Verification items for this drawing (mm, ordinates from the low corner). A direction names the side the tool comes from. Coordinates: 2 decimals unless noted, no trailing zeros. Write each loop counter-clockwise with the first axis right and the second up, starting at its lowest first coordinate (ties: lowest second). Pieces come first, ordered by that corner, then holes. Notation, with made-up numbers: (87, 87.25) -> (129, 87.25) arc R8 cw to (129, 96.25) -> close; hole circle Ø8 at (78.25, 31.25). An arc over 180 degrees is marked (long way). One line per question, with ' | ' between items.
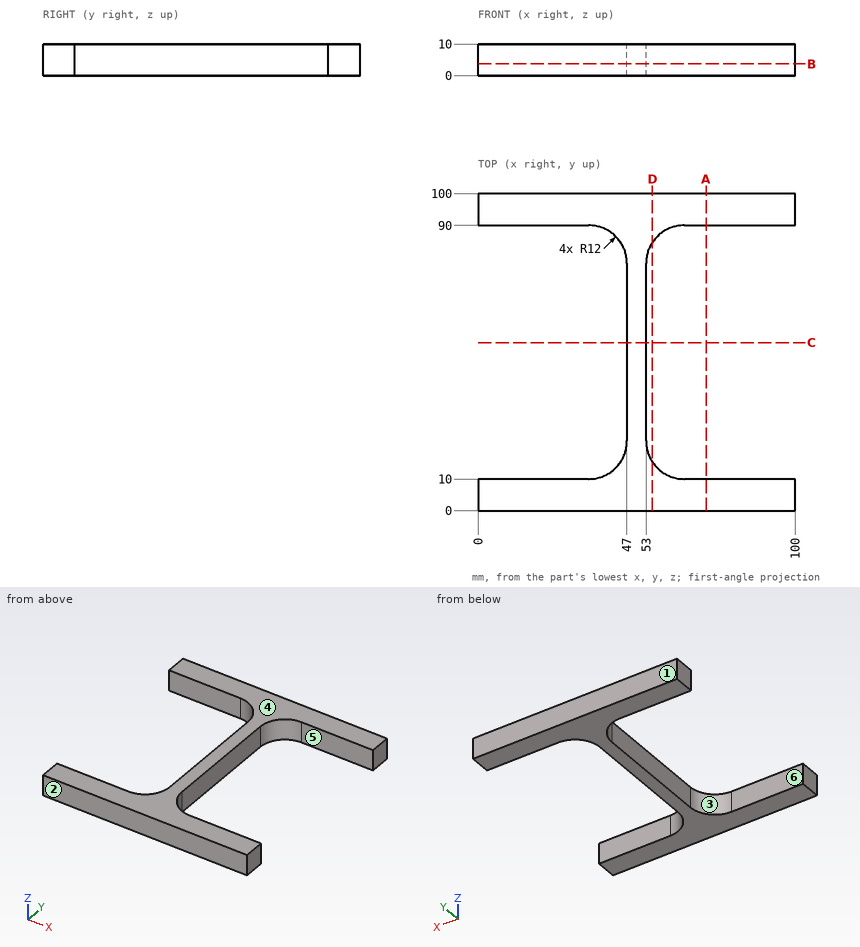
(1) Cross-section at D-D (x = 55). Record the cut outline in (y, z), plus the area to 3 significant figures.
Answers below:
outline: (0, 0) -> (15.37, 0) -> (15.37, 10) -> (0, 10) -> close; (84.63, 0) -> (100, 0) -> (100, 10) -> (84.63, 10) -> close | area: 307 mm²
(2) Material ranges on line 1 (Y direction, x = 71.5, z = 9.75); line 2 (X direction, y = 25, z = 9.75); line 3 (X direction, y = 20, z = 6.75), recorded low to high.
Answers below:
line 1: y = 0 to 10, 90 to 100 | line 2: x = 47 to 53 | line 3: x = 46.83 to 53.17
(3) Depth check by flat-ended pin: P1, Ø5, axis at y = 78, z = 6, coming from the -X side. Enter the tip coordinate at first touch or a pass-through.
Answers below:
P1: stops at x = 46.74
(4) Draft check along Y on the marked faces 1, 2 and 3. Enter one of: pulls with the +Y half, pulls with the -Y half, needs draft (parallel to the pull), parting line crosses it, or undercut.
Answers below:
face 1: pulls with the +Y half | face 2: pulls with the -Y half | face 3: undercut
(5) Cross-section at B-B (z = 3.75). Record the cut outline in (x, y).
Answers below:
outline: (0, 0) -> (100, 0) -> (100, 10) -> (65, 10) arc R12 cw to (53, 22) -> (53, 78) arc R12 cw to (65, 90) -> (100, 90) -> (100, 100) -> (0, 100) -> (0, 90) -> (35, 90) arc R12 cw to (47, 78) -> (47, 22) arc R12 cw to (35, 10) -> (0, 10) -> close
(6) Tool access check on the marked faces 4, 5 and 6. Record the directions out of +Z, -Z, +X, -X, +Y, -Y that give a thin tool (end or side, any length) a straight path to the whole face; none if there is none.
Answers below:
face 4: +Z, +X, -X, +Y, -Y | face 5: +Z, -Z, +X | face 6: +Z, -Z, -X
(7) Cross-section at A-A (x = 72). Record the cut outline in (y, z), plus the area to 3 significant figures.
Answers below:
outline: (0, 0) -> (10, 0) -> (10, 10) -> (0, 10) -> close; (90, 0) -> (100, 0) -> (100, 10) -> (90, 10) -> close | area: 200 mm²
(8) Cross-section at C-C (y = 53). Record the cut outline in (x, z), plus the area to 3 significant figures.
Answers below:
outline: (47, 0) -> (53, 0) -> (53, 10) -> (47, 10) -> close | area: 60.0 mm²
